The drawing under review shows one solid part. Ordinate dimensions are in mm from its lowest x, y, z. Coordinates: 2 decimals unless noted, no trailing zeros. Order: outer loops, then holes, each group sorted by start corner. A loop starts at its lowest first (then second) coordinate and runs counter-clockwise, first axis right, second up. Notation, with made-up numbers: (-28, 17.5) -> (-16, 17.5) arc R20 ccw to (-16, 25.5) -> close; hole circle Ø4 at (-37, 22.5). An arc over 180 degrees is marked (long way). Put each result on its own line as item: value.
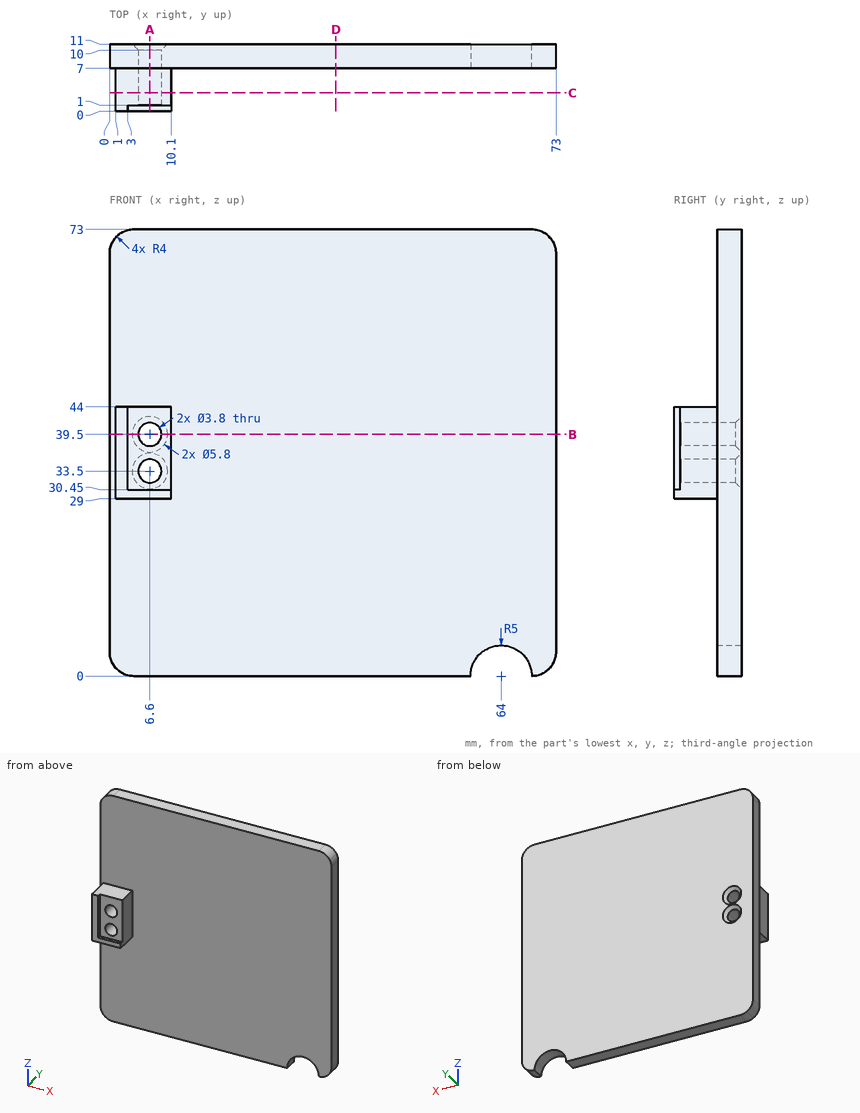
Item 1: Consider section A-A on x = 6.6. Write out the cut boundary in (y, z), and give its area (3 significant figures).
Answers below:
outline: (0, 29) -> (7, 29) -> (7, 0) -> (11, 0) -> (11, 30.6) -> (10, 31.6) -> (1, 31.6) -> (1, 30.45) -> (0, 30.45) -> close; (1, 35.4) -> (10, 35.4) -> (11, 36.4) -> (11, 36.6) -> (10, 37.6) -> (1, 37.6) -> close; (1, 41.4) -> (10, 41.4) -> (11, 42.4) -> (11, 73) -> (7, 73) -> (7, 44) -> (1, 44) -> close
area: 305 mm^2
Item 2: Consider section C-C on y = 3. Write out the cut boundary in (x, z).
Answers below:
outline: (1, 29) -> (10.1, 29) -> (10.1, 44) -> (1, 44) -> close; hole circle Ø3.8 at (6.6, 33.5); hole circle Ø3.8 at (6.6, 39.5)
Item 3: Consider section D-D on x = 37. Write out the cut boundary in (y, z), and give its area (3 significant figures).
Answers below:
outline: (7, 0) -> (11, 0) -> (11, 73) -> (7, 73) -> close
area: 292 mm^2
Item 4: For pin 1 Ø0.8 at (x, y) = (6, 0.5) entering from +Z; pin 2 Ø2 at (x, z) = (5, 36.5) entering from -Y; pin 3 Ø4 at (x, z) = (11, 60.5) entering from -Y, all flat-tipped, find the tip position at first contact; note any pin that passes through.
Answers below:
pin 1: z = 30.45
pin 2: y = 1
pin 3: y = 7
Item 5: For line 1 (Z direction, x = 6.6, y = 4); line 2 (Z direction, x = 6.6, y = 7.5); line 3 (Y direction, x = 21, z = 26.5), list the stretches that pass through material, from the lowest coordinate up. Write a range as from..to.
Answers below:
line 1: 29..31.6, 35.4..37.6, 41.4..44
line 2: 0..31.6, 35.4..37.6, 41.4..73
line 3: 7..11
Item 6: Consider section B-B on z = 39.5. Write out the cut boundary in (x, y), and give its area (3 significant figures).
Answers below:
outline: (0, 7) -> (1, 7) -> (1, 0) -> (3, 0) -> (3, 1) -> (4.7, 1) -> (4.7, 10) -> (3.7, 11) -> (0, 11) -> close; (8.5, 1) -> (10.1, 1) -> (10.1, 7) -> (73, 7) -> (73, 11) -> (9.5, 11) -> (8.5, 10) -> close
area: 310 mm^2
